```python
from build123d import *

# Parameters (mm, degrees)
SKETCH_1_R          = 8
EXTRUDE_1_DEPTH     = 18.7
SKETCH_2_W          = 4
SKETCH_2_H          = 6
CUT_EXTRUDE_1_DEPTH = 18.7
OTHER_START         = 9.35
OTHER_4_OUTLINE_R   = 8
OTHER_4_OUTLINE_R_2 = 4.714576893
OTHER_4_DEPTH       = 0.65
SKETCH_1_3_R        = 0.85
CUT_EXTRUDE_2_DEPTH = 2
CUT_EXTRUDE_START   = 16.7
SKETCH_1_4_R        = 0.85
CUT_EXTRUDE_3_DEPTH = 2
SKETCH_1_6_R        = 0.85
CUT_EXTRUDE_4_DEPTH = 2
SKETCH_1_7_R        = 0.85
CUT_EXTRUDE_5_DEPTH = 2


# Read off the part's stored shape, not the designer's step: 切除-旋转-薄壁4
with BuildPart() as part:
    # 草图1 → 凸台-拉伸1 (new body)
    with BuildSketch(Plane.XY):
        Circle(SKETCH_1_R)
    extrude(amount=EXTRUDE_1_DEPTH)

    # 草图2 → 切除-拉伸1 (cut)
    with BuildSketch(Plane(origin=(0, 0, 0), x_dir=(0, 0, -1), z_dir=(1, 0, 0))):
        with Locations((-13.9, 0)):
            Rectangle(SKETCH_2_W, SKETCH_2_H)
    extrude(amount=-CUT_EXTRUDE_1_DEPTH, mode=Mode.SUBTRACT)

    # 切除-旋转-薄壁4 outline → 切除-旋转-薄壁4 (cut)
    with BuildSketch(Plane.XY.offset(OTHER_START)):
        Circle(OTHER_4_OUTLINE_R)
        Circle(OTHER_4_OUTLINE_R_2, mode=Mode.SUBTRACT)
    extrude(amount=OTHER_4_DEPTH, mode=Mode.SUBTRACT)

    # 草图1<3> → 切除-拉伸2 (cut)
    with BuildSketch(Plane.XY):
        with Locations((-6, 0)):
            Circle(SKETCH_1_3_R)
        with Locations((3, 5.196152423)):
            Circle(SKETCH_1_3_R)
    extrude(amount=CUT_EXTRUDE_2_DEPTH, mode=Mode.SUBTRACT)

    # 草图1<4> → 切除-拉伸3 (cut)
    with BuildSketch(Plane.XY.offset(CUT_EXTRUDE_START)):
        with Locations((-6, 0)):
            Circle(SKETCH_1_4_R)
        with Locations((3, 5.196152423)):
            Circle(SKETCH_1_4_R)
    extrude(amount=CUT_EXTRUDE_3_DEPTH, mode=Mode.SUBTRACT)

    # 草图1<6> → 切除-拉伸4 (cut)
    with BuildSketch(Plane.XY):
        with Locations(Location((3, -5.196152423, 0), (0, 0, 180))):
            Circle(SKETCH_1_6_R)
    extrude(amount=CUT_EXTRUDE_4_DEPTH, mode=Mode.SUBTRACT)

    # 草图1<7> → 切除-拉伸5 (cut)
    with BuildSketch(Plane.XY.offset(CUT_EXTRUDE_START)):
        with Locations(Location((3, -5.196152423, 0), (0, 0, 180))):
            Circle(SKETCH_1_7_R)
    extrude(amount=CUT_EXTRUDE_5_DEPTH, mode=Mode.SUBTRACT)


solid = part.part
```
Can you work these out from the model? Positions are in its coordinate system, mm. A direction names the side the tool comes from. Give positions to 0.01 mm unless a question says otherwise; leave off trailing zeros. Order: outer loops, then holes, each group sorted by start corner. A loop starts at its lowest first (then second) coordinate and runs counter-clockwise, first axis right, second up. Notation, with made-up numbers: (-10.75, 87.25) - (28.25, 87.25) arc R19 cw to (28.25, 97.25) - close; hole circle Ø9 at (-6.75, 39.5). An arc over 180 degrees is marked (long way). Use a Markdown table: item, result. Add a question column.
Q1. If we section it at B-B on y = 0: Write out the boundary of the cut face in (x, z), plus the area to 3 significant figures.
Q2. If we section it at C-C on x = 6.25: Write out the boundary of the cut face in (y, z), plus the area to 3 significant figures.
Q3. If we mould it in two halves opening along Z, with no side actions, what happens to faces 1 (the flat face through (-6, 0, 16.7)), 2 (the cylindrical face through (3.11, -6.04, 17.69)), 3 (the flat face through (-4, 3, 14)), 4 (the flat face through (0, 0, 14))? For each: released by +Z, released by -Z, zero draft, split by the parting line, or undercut.
Q4. If we section it at D-D on x = -0.75: Write out the boundary of the cut face in (y, z), plus the area to 3 significant figures.
Q5. If we section it at A-A on x = -6: Write out the boundary of the cut face in (y, z).
Q6. On a 3-axis mill with a long thin cutter (end or side, diameter ignored), from which of +Z, -Z, +X, -X, +Y, -Y can I reach the whole of each face in a straight line? I mean faces 5 (the flat face through (3.44, -3.44, 10)), 6 (the flat face through (3, 5, 16.7)), 7 (the flat face through (-6, 0, 2)), 8 (the flat face through (-4, 0, 15.9)). Say none if no direction works.
Q7. I'm going to push flat-ended pins straight in: pin 1 (2 mm diameter, centred on x = -2, z = 14.5, fed in from +Y); pin 2 (1.4 mm diameter, centred on x = -6, y = 0, fed in from +Z); pin 3 (4 mm diameter, centred on y = 6, z = 2.5, fed in from +X). Where does each tip first touch, or does it pass through?
Q8. Please list where these lines run through material, in increasing order: line 1 along Z through (x, y) = (-5, 4); line 2 along Y through (x, z) = (3, 1.45); line 3 along Y through (x, z) = (-0.75, 15.5).
Answers follow:
| question | item | result |
|---|---|---|
| 1 | outline | (-8, 0) - (-6.85, 0) - (-6.85, 2) - (-5.15, 2) - (-5.15, 0) - (8, 0) - (8, 9.35) - (4.71, 9.35) - (4.71, 10) - (8, 10) - (8, 18.7) - (-5.15, 18.7) - (-5.15, 16.7) - (-6.85, 16.7) - (-6.85, 18.7) - (-8, 18.7) - (-8, 15.9) - (0, 15.9) - (0, 11.9) - (-8, 11.9) - (-8, 10) - (-4.71, 10) - (-4.71, 9.35) - (-8, 9.35) - close |
| 1 | area | 256 mm^2 |
| 2 | outline | (-4.99, 0) - (4.99, 0) - (4.99, 9.35) - (-4.99, 9.35) - close; (-4.99, 10) - (4.99, 10) - (4.99, 18.7) - (-4.99, 18.7) - close |
| 2 | area | 180 mm^2 |
| 3 | face 1 | released by +Z |
| 3 | face 2 | zero draft |
| 3 | face 3 | undercut |
| 3 | face 4 | undercut |
| 4 | outline | (-7.96, 0) - (7.96, 0) - (7.96, 9.35) - (4.65, 9.35) - (4.65, 10) - (7.96, 10) - (7.96, 18.7) - (-7.96, 18.7) - (-7.96, 10) - (-4.65, 10) - (-4.65, 9.35) - (-7.96, 9.35) - close; hole (-3, 11.9) - (3, 11.9) - (3, 15.9) - (-3, 15.9) - close |
| 4 | area | 270 mm^2 |
| 5 | outline | (-5.29, 0) - (-0.85, 0) - (-0.85, 2) - (0.85, 2) - (0.85, 0) - (5.29, 0) - (5.29, 9.35) - (-5.29, 9.35) - close; (-5.29, 10) - (5.29, 10) - (5.29, 18.7) - (0.85, 18.7) - (0.85, 16.7) - (-0.85, 16.7) - (-0.85, 18.7) - (-5.29, 18.7) - close; hole (-3, 11.9) - (3, 11.9) - (3, 15.9) - (-3, 15.9) - close |
| 6 | face 5 | none |
| 6 | face 6 | +Z |
| 6 | face 7 | -Z |
| 6 | face 8 | -X |
| 7 | pin 1 | stops at y = 7.94 |
| 7 | pin 2 | stops at z = 16.7 |
| 7 | pin 3 | stops at x = 6.93 |
| 8 | line 1 | z = 0 to 9.35, 10 to 18.7 |
| 8 | line 2 | y = -7.42 to -6.05, -4.35 to 4.35, 6.05 to 7.42 |
| 8 | line 3 | y = -7.96 to -3, 3 to 7.96 |
